Autodesk Fusion 360 part; units mm, degrees
sketch "Sketch1" plane through (0, 0, 0) normal (0, 1, 0) x (1, 0, 0)
  circle A0 centre (0, 0) radius 3.55
  circle A1 centre (0, 0) radius 6
  dimension "d1" = 7.1
  dimension "d2" = 12
extrude "Extrude1" add sketch "Sketch1" against normal blind 5
sketch "Sketch2" plane through (0, 0, 0) normal (0, 1, 0) x (-1, 0, 0)
  circle A0 centre (0, 0) radius 3.55
  circle A1 centre (0, 0) radius 6
  circle A2 centre (0, 0) radius 8.5
  dimension "d5" = 17
extrude "Extrude2" add sketch "Sketch2" along normal blind 3 contours A0 | A1 | A2
sketch "Sketch3" plane through (0, 3, 0) normal (0, 1, 0) x (-1, 0, 0)
  circle A0 centre (0, 0) radius 8.5
  circle A1 centre (0, 0) radius 6
  dimension "d8" = 12
extrude "Extrude3" add sketch "Sketch3" along normal blind 5 contours A1
sketch "Sketch4" plane through (0, 8, 0) normal (0, 1, 0) x (-1, 0, 0)
  circle A0 centre (0, 0) radius 6
  circle A1 centre (0, 0) radius 8.5
extrude "Extrude4" add sketch "Sketch4" along normal blind 3 contours A0 | A1
sketch "Sketch5" plane through (0, 0, 0) normal (1, 0, 0) x (0, 0, -1)
  circle A0 centre (0, 5) radius 1.5
  dimension "d13" = 3
extrude "Extrude5" cut sketch "Sketch5" along normal blind 10 and the other way blind 12
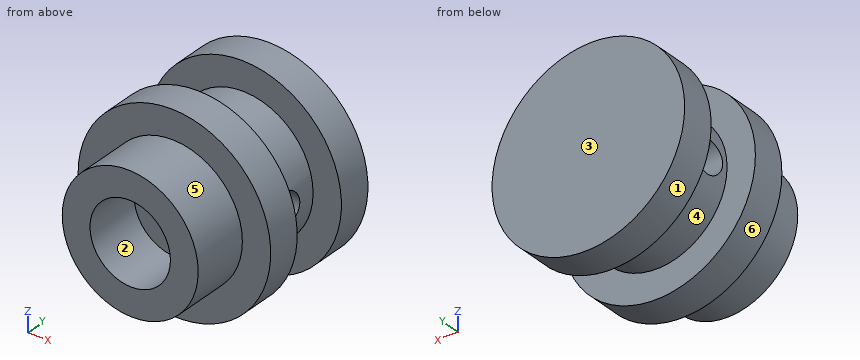
Work out the finished part from the listing and answer in its coordinate system (mm). Face numbers are marked on the shaded views. A direction names the side the tool comes from. Give positions to 0.01 mm unless a question says otherwise; leave off trailing zeros. Write each loop counter-clockwise with the first axis right and the second up, starting at its lowest first coordinate (ties: lowest second). Pieces come first, ordered by that corner, then holes.
Q1. The part is cut by section C-C on x = -6.75. Give the vertices of the cut face in (y, z).
Answer:
outline: (0, -5.17) - (3, -5.17) - (3, 5.17) - (0, 5.17) - close; (8, -5.17) - (11, -5.17) - (11, 5.17) - (8, 5.17) - close
Q2. Straight lines are drawn through the part: L1, parallel to Y at x = 6.75, z = 4.5; L2, parallel to X at y = -1.7, z = 0. For each, find the intervals that lie inside material, in ascending order.
Answer:
L1: y = 0 to 3, 8 to 11
L2: x = -6 to -3.55, 3.55 to 6
Q3. For a pull along X with two mould halves and no side action, classify the marked faces 1, 2 and 3 as released by +X, released by -X, zero draft, split by the parting line, or undercut.
Answer:
face 1: split by the parting line
face 2: undercut
face 3: zero draft
Q4. The part is cut by section A-A on x = 0. Give the vertices of the cut face in (y, z).
Answer:
outline: (-5, -6) - (0, -6) - (0, -8.5) - (3, -8.5) - (3, -6) - (8, -6) - (8, -8.5) - (11, -8.5) - (11, 8.5) - (8, 8.5) - (8, 6) - (3, 6) - (3, 8.5) - (0, 8.5) - (0, 6) - (-5, 6) - (-5, 3.55) - (0, 3.55) - (0, -3.55) - (-5, -3.55) - close; hole circle Ø3 at (5, 0)
Q5. A tool of negligible diameter and unlimited length cuts with its end or side. For the marked faces 4, 5 and 6, from which of +Z, -Z, +X, -X, +Y, -Y can it reach the whole face along a straight path? Write none if from no direction.
Answer:
face 4: none
face 5: -Y
face 6: +Y, -Y
Q6. The part is cut by section B-B on z = 6.5. Give the vertices of the cut face in (x, y), and give its area (3 significant figures).
Answer:
outline: (-5.48, 0) - (5.48, 0) - (5.48, 3) - (-5.48, 3) - close; (-5.48, 8) - (5.48, 8) - (5.48, 11) - (-5.48, 11) - close
area: 65.7 mm2
Q7. The part is cut by section D-D on y = -2.5. Give the vertices of the cut face in (x, z), and give its area (3 significant figures).
Answer:
outline: circle Ø12 at (0, 0); hole circle Ø7.1 at (0, 0)
area: 73.5 mm2
Q8. Given pin 1 (3 mm diameter, centred on x = 4.5, y = 6, fed in from +Z); pin 2 (2 mm diameter, centred on x = -1.5, z = 0.5, fed in from -Y), each flat-ended and moving along its own axis, determine where each tip first touches the part or whether it passes through.
Answer:
pin 1: stops at z = 5.2
pin 2: stops at y = 0
